Geometry: final body of the model. Coordinates: model frame, mm. Face numbers are marked on the shaded views. A direction names the side the tool comes from. Coordinates: 2 decimals unless noted, no trailing zeros. Order: outer loops, then holes, each group sorted by start corner. A loop starts at its lowest first (then second) coordinate and runs counter-clockwise, first axis right, second up. Notation, with made-up numbers: M -27.75,61 L -0.75,61 A20 ccw -0.75,82 Z; hole C 61.25,83 d10. An arc over 180 degrees is marked long. Write item = value, one per line.
from build123d import *

# Parameters (mm, degrees)
SKETCH_1_R          = 14.149308539
SKETCH_1_R_2        = 1.6
EXTRUDE_1_DEPTH     = 4
EXTRUDE_2_DEPTH     = 10
CUT_EXTRUDE_START   = -10
SKETCH_4_R          = 1.6
CUT_EXTRUDE_1_DEPTH = 10


with BuildPart() as part:
    # 草图1 → 凸台-拉伸1 (new body)
    with BuildSketch(Plane.XY):
        Circle(SKETCH_1_R)
        with Locations((0, -8)):
            Circle(SKETCH_1_R_2, mode=Mode.SUBTRACT)
        with Locations((8, 0)):
            Circle(SKETCH_1_R_2, mode=Mode.SUBTRACT)
        with Locations((0, 8)):
            Circle(SKETCH_1_R_2, mode=Mode.SUBTRACT)
        with Locations((-8, 0)):
            Circle(SKETCH_1_R_2, mode=Mode.SUBTRACT)
    extrude(amount=EXTRUDE_1_DEPTH)

    # 草图3 → 凸台-拉伸2 (add)
    with BuildSketch(Plane(origin=(0, 0, 0), x_dir=(0, 0, -1), z_dir=(0.7071067811865488, 0.7071067811865464, 0))):
        with BuildLine():
            Line((-8, 9), (-8, 2))
            ThreePointArc((-8, 2), (-6.585786438, 1.414213562), (-6, 0))
            ThreePointArc((-6, 0), (-6.585786438, -1.414213562), (-8, -2))
            Line((-8, -2), (-8, -9))
            Line((-8, -9), (-4, -9))
            Line((-4, -9), (-4, 9))
            Line((-4, 9), (-8, 9))
        make_face()
    extrude(amount=EXTRUDE_2_DEPTH)

    # 草图4 → 切除-拉伸1 (cut)
    with BuildSketch(Plane.XY.offset(8).offset(CUT_EXTRUDE_START)):
        with Locations((8, 0)):
            Circle(SKETCH_4_R)
        with Locations((0, 8)):
            Circle(SKETCH_4_R)
    extrude(amount=CUT_EXTRUDE_1_DEPTH, mode=Mode.SUBTRACT)


solid = part.part
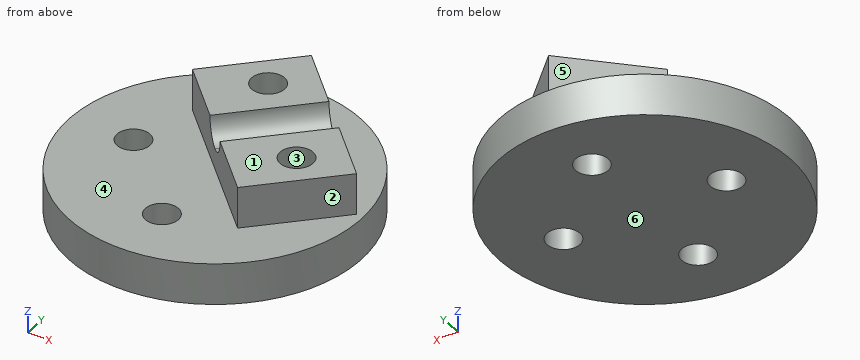
1) Section D-D, the plane x = 10.75. Return loops of the section in (y, z).
Numbers:
outline = M -9.2,0 L 9.2,0 L 9.2,4 L 3.39,4 L 3.39,8 L -1.98,8 L -1.98,4 L -9.2,4 Z
2) Line query: L1, parallel to Y at x = 0, z = 1.1; L2, parallel to X at y = -0.5, z = 0.5; L3, parallel to Z at x = 4.5, y = 11.75. Output: solid intervals per line, ascending.
Numbers:
L1 = -14.15 to -9.6, -6.4 to 6.4, 9.6 to 14.15
L2 = -14.14 to -9.52, -6.48 to 6.48, 9.52 to 14.14
L3 = 0 to 4
3) Mould query, pull axis X, two halves, no side actions, for the marked faces 1, 2 and 3. Classes: pulls with the +X half, pulls with the -X half, needs draft (parallel to the pull), parting line crosses it, or undercut.
Numbers:
face_1 = needs draft
face_2 = pulls with the +X half
face_3 = undercut
4) Section A-A, the plane y = -8. Return loops of the section in (x, z), and give its area (3 significant figures).
Numbers:
outline = M -11.67,0 L -1.6,0 L -1.6,4 L -11.67,4 Z; M 1.6,0 L 11.67,0 L 11.67,4 L 1.6,4 Z
area = 80.6 mm²
5) Set-up query: the marked faces 4, 5 and 6. Return all of +Z, -Z, +X, -X, +Y, -Y with unobstructed straight access to the full face (end or side cutting, diameter ignored); none if empty.
Numbers:
face_4 = +Z
face_5 = +Z, -X, +Y
face_6 = -Z, +X, -X, +Y, -Y
6) Section B-B, the plane z = 3.25. Return loops of the section in (x, y), and give its area (3 significant figures).
Numbers:
outline = C 0,0 d28.3; hole C -8,0 d3.2; hole C 0,-8 d3.2; hole C 0,8 d3.2; hole C 8,0 d3.2
area = 597 mm²
7) Pin query (flat end, axial travel): pin 1 (2 mm diameter, centred on x = -5.5, y = -9.5, fed in from +Z); pin 2 (1.9 mm diameter, centred on x = 8, y = 0, fed in from +Z); pin 3 (2 mm diameter, centred on x = 2, z = 6.5, fed in from +Y); pin 4 (4 mm diameter, centred on x = 3, z = 5.5, fed in from +Y). Return the tip coordinate at first contact, or that it passes through.
Numbers:
pin_1 = 4
pin_2 = through
pin_3 = 13.14
pin_4 = 14.05
